CAD build for the part. Positions are in the model's coordinates, mm. A direction names the side the tool comes from. Give positions to 0.01 mm unless a question says otherwise; leave off trailing zeros. Write each loop counter-clockwise with the first axis right and the second up, starting at its lowest first coordinate (ties: lowest second). Pieces come first, ordered by that corner, then holes. Notation, with made-up numbers: (-31.75, 56.5) -> (23.25, 56.5) arc R11 cw to (23.25, 75.5) -> close; hole circle Ø4 at (-11, -38.75). An arc over 180 degrees is marked (long way). Answer in a Markdown table with one row per item. Add a question column.
```python
from build123d import *

# Parameters (mm, degrees)
F1_DEPTH      = 2.54
F3_DEPTH      = 76.2
F4_W          = 16.2733292935
F4_H          = 18.6266666667
F4_W_2        = 0.444823617
F5_DEPTH      = 3.6743734411
F5_DEPTH_BACK = 6.4876265589


with BuildPart() as f1:
    # F0 (on Top) → F1 (new body)
    with BuildSketch(Plane.XY):
        with BuildLine():
            Line((0, 76.2), (0, 0))
            Line((0, 0), (20.32, 0))
            ThreePointArc((20.32, 0), (33.7903841816, 5.5796158184), (39.37, 19.05))
            Line((39.37, 19.05), (39.37, 57.15))
            ThreePointArc((39.37, 57.15), (33.7903841816, 70.6203841816), (20.32, 76.2))
            Line((20.32, 76.2), (0, 76.2))
        make_face()
    extrude(amount=F1_DEPTH)

    # F2 (on face) → F3 (join, through all)
    with BuildSketch(Plane.XZ):
        with BuildLine():
            Line((0, 2.54), (-0.444823617, 2.54))
            ThreePointArc((-0.444823617, 2.54), (-9.5610605276, 6.7523933173), (-2.1276752047, 0))
            Line((-2.1276752047, 0), (0, 0))
            Line((0, 0), (0, 2.54))
        make_face()
    extrude(amount=-F3_DEPTH)

    # F4 (on face) → F5 (cut, two sides)
    with BuildSketch(Plane.XY.offset(2.54)) as f5_sk:
        with Locations((-8.5814882637, 56.7266666667)):
            Rectangle(F4_W, F4_H)
        with Locations((-0.2224118085, 56.7266666667)):
            Rectangle(F4_W_2, F4_H)
        with Locations((-8.5814882637, 19.4733333333)):
            Rectangle(F4_W, F4_H)
        with Locations((-0.2224118085, 19.4733333333)):
            Rectangle(F4_W_2, F4_H)
    extrude(amount=-F5_DEPTH, mode=Mode.SUBTRACT)
    extrude(f5_sk.sketch, amount=F5_DEPTH_BACK, mode=Mode.SUBTRACT)


solid = f1.part
```
Item 1: Mould opens along Y. For faces 4 (the face through (-5, 28.787, 4)), 5 (the face through (-2, 0, 3)), 6 (the face through (-2, 76.2, 3)), 7 (the face through (0, 57, 1)) say: released by +Y, released by -Y, zero draft, split by the parting line, or undercut.
Item 2: Drop flat-ended pins along their axis: pin 1 Ø3 at (x, z) = (30.5, 2) entering from +Y; pin 2 Ø5 at (y, z) = (52, 0.5) entering from -X; pin 3 Ø10 at (x, y) = (32, 33.5) entering from -Z; pin 4 Ø12 at (x, y) = (-1, 65) entering from +Z. Give the stop position or say it passes through.
Item 3: Slice it at C-C, the plane z = 1.5. List the corners of the cut face in (x, y), then the cut area to 3 significant figures.
Item 4: Slice it at D-D, the plane x = 16. List the corners of the cut face in (y, z), then the cut area to 3 significant figures.
Item 5: Which spindle directions (+Z, -Z, +X, -X, +Y, -Y) get a long thin tool onto all of the face, cutting with end or side? Do faces 1 (the face through (-5, 47.413, 4)), 2 (the face through (33.64, 5.43, 1.25)), 3 (the face through (18, 38, 0)). Say none if no direction does.
Item 6: Slice it at A-A, the plane z = 5.25. List the corners of the cut face in (x, y).
Item 7: Slice it at B-B, the plane y = 32.5. List the corners of the cut face in (x, z), then the cut area to 3 significant figures.
Item 8: Probe L1, parallel to Y at x = -8, z = -0.25; L2, parallel to Z at x = 24, y = 57.5; L3, parallel to X at y = 67.5, z = 4.25. List the from-to ranges inside material, lowest first. Write a range as from..to.
Answer key:
| question | item | result |
|---|---|---|
| 1 | face 4 | undercut |
| 1 | face 5 | released by -Y |
| 1 | face 6 | released by +Y |
| 1 | face 7 | undercut |
| 2 | pin 1 | stops at y = 74.11 |
| 2 | pin 2 | stops at x = 0 |
| 2 | pin 3 | stops at z = 0 |
| 2 | pin 4 | stops at z = 9.03 |
| 3 | outline | (-9.78, 0) -> (20.32, 0) arc R19.05 ccw to (39.37, 19.05) -> (39.37, 57.15) arc R19.05 ccw to (20.32, 76.2) -> (-9.78, 76.2) -> (-9.78, 66.04) -> (0, 66.04) -> (0, 47.41) -> (-9.78, 47.41) -> (-9.78, 28.79) -> (0, 28.79) -> (0, 10.16) -> (-9.78, 10.16) -> close |
| 3 | area | 3,230 mm² |
| 4 | outline | (0, 0) -> (76.2, 0) -> (76.2, 2.54) -> (0, 2.54) -> close |
| 4 | area | 194 mm² |
| 5 | face 1 | +Z, -Z, -X |
| 5 | face 2 | +Z, -Z, +X, -Y |
| 5 | face 3 | -Z, +X, +Y, -Y |
| 6 | outline | (-10.24, 0) -> (-0.42, 0) -> (-0.42, 10.16) -> (-10.24, 10.16) -> close; (-10.24, 28.79) -> (-0.42, 28.79) -> (-0.42, 47.41) -> (-10.24, 47.41) -> close; (-10.24, 66.04) -> (-0.42, 66.04) -> (-0.42, 76.2) -> (-10.24, 76.2) -> close |
| 7 | outline | (-2.13, 0) -> (39.37, 0) -> (39.37, 2.54) -> (-0.44, 2.54) arc R5.08 ccw (long way) to start |
| 7 | area | 184 mm² |
| 8 | L1 | y = 0..10.16, 28.79..47.41, 66.04..76.2 |
| 8 | L2 | z = 0..2.54 |
| 8 | L3 | x = -10.4..-0.26 |
